Input: part model. Units: mm. Frame: model coordinates. A direction names the side the tool comes from. Round coordinates to 2 decimals unless told otherwise and drop trailing zeros. Loops run counter-clockwise (first coordinate to the right, second up) from the corner with the lowest first, then second, coordinate; pieces in that order, holes last. Notation, with made-up numbers: (-33, -21) -> (25, -21) arc R12 ccw to (25, -15) -> close; hole circle Ø8 at (-2, 26.25). An arc over 180 degrees is marked (long way). Answer as a JSON object with one key per item and string values. Group by question number.
Item 1: Section query B-B on x = -26. Return loops of the section in (y, z), and give its area (3 significant figures).
Item 2: Material intervals for line 1 (Y direction, x = 20.5, z = 4); line 2 (X direction, y = -8, z = 4.25); line 3 (X direction, y = -22.5, z = 17), sorted ascending. Write a range as [from, to].
Item 3: Section query A-A on y = 9. Return loops of the section in (x, z), and give its area (3 significant figures).
Item 4: Draft query along X for faces 3 (the cylindrical face through (-36.19, 29.94, 12.52)), 4 (the cylindrical face through (37.742, 27.501, 12.522)), 5 (the flat face through (0, 29.21, 13)), 6 (the flat face through (0, -29.21, 13)). Return one class per face: released by +X, released by -X, zero draft, split by the parting line, or undercut.
Item 5: Set-up query: faces 1 (the flat face through (-35.56, 1, 13)), 2 (the cylindrical face through (36.19, -29.94, 12.52)). Return all of +Z, -Z, +X, -X, +Y, -Y with unobstructed straight access to the full face (end or side cutting, diameter ignored); none if empty.
from build123d import *

# Parameters (mm, degrees)
F1_DEPTH = 25.4
F2_T     = -2.54
F4_DEPTH = 25.4


with BuildPart() as f1:
    # F0 (on Top) → F1 (new body)
    with BuildSketch(Plane.XY):
        with BuildLine():
            Line((-31.75, -31.75), (31.75, -31.75))
            ThreePointArc((31.75, -31.75), (36.2401280605, -29.8901280605), (38.1, -25.4))
            Line((38.1, -25.4), (38.1, 25.4))
            ThreePointArc((38.1, 25.4), (36.2401280605, 29.8901280605), (31.75, 31.75))
            Line((31.75, 31.75), (-31.75, 31.75))
            ThreePointArc((-31.75, 31.75), (-36.2401280605, 29.8901280605), (-38.1, 25.4))
            Line((-38.1, 25.4), (-38.1, -25.4))
            ThreePointArc((-38.1, -25.4), (-36.2401280605, -29.8901280605), (-31.75, -31.75))
        make_face()
    extrude(amount=F1_DEPTH)

    # F2
    f2_openings = [f1.faces().sort_by_distance(p)[0] for p in [
        (0, 0, 0),
        (0, 0, 25.4),
    ]]
    offset(amount=F2_T, openings=f2_openings)

    # F3 (on Top) → F4 (join)
    with BuildSketch(Plane.XY):
        with BuildLine():
            ThreePointArc((-34.8345838171, 24.6476917684), (-31.3711389564, 22.2476850872), (-28.575, 25.4))
            ThreePointArc((-28.575, 25.4), (-29.2094457266, 27.3042607447), (-30.8592261315, 28.4474820615))
            ThreePointArc((-30.8592261315, 28.4474820615), (-30.7914950358, 28.0740348735), (-30.7688099486, 27.6951738299))
            ThreePointArc((-30.7688099486, 27.6951738299), (-32.0395492039, 25.1546195565), (-34.8345838171, 24.6476917684))
        make_face()
        with BuildLine():
            ThreePointArc((-30.7688099486, 27.6951738299), (-30.7914950358, 28.0740348735), (-30.8592261315, 28.4474820615))
            ThreePointArc((-30.8592261315, 28.4474820615), (-33.9438099486, 27.6951738299), (-34.8345838171, 24.6476917684))
            ThreePointArc((-34.8345838171, 24.6476917684), (-32.0395492039, 25.1546195565), (-30.7688099486, 27.6951738299))
        make_face()
        with BuildLine():
            ThreePointArc((-34.8345838171, 24.6476917684), (-33.9438099486, 27.6951738299), (-30.8592261315, 28.4474820615))
            ThreePointArc((-30.8592261315, 28.4474820615), (-36.1376198972, 29.9903476598), (-34.8345838171, 24.6476917684))
        make_face()
        with BuildLine():
            ThreePointArc((-31.75, -28.575), (-29.5049359697, -27.6450640303), (-28.575, -25.4))
            ThreePointArc((-28.575, -25.4), (-30.5019458319, -22.480584683), (-33.9438099486, -23.1048261701))
            ThreePointArc((-33.9438099486, -23.1048261701), (-31.6987459183, -24.0347621398), (-30.7688099486, -26.2798261701))
            ThreePointArc((-30.7688099486, -26.2798261701), (-31.0243946315, -27.5278803382), (-31.75, -28.575))
        make_face()
        with BuildLine():
            ThreePointArc((-30.7688099486, -26.2798261701), (-31.6987459183, -24.0347621398), (-33.9438099486, -23.1048261701))
            ThreePointArc((-33.9438099486, -23.1048261701), (-34.6968459334, -26.5818308022), (-31.75, -28.575))
            ThreePointArc((-31.75, -28.575), (-31.0243946315, -27.5278803382), (-30.7688099486, -26.2798261701))
        make_face()
        with BuildLine():
            ThreePointArc((-31.75, -28.575), (-34.6968459334, -26.5818308022), (-33.9438099486, -23.1048261701))
            ThreePointArc((-33.9438099486, -23.1048261701), (-36.890655882, -27.4616569723), (-31.75, -28.575))
        make_face()
        with BuildLine():
            ThreePointArc((34.8303002747, 24.630340843), (34.9012361362, 25.0122683738), (34.925, 25.4))
            ThreePointArc((34.925, 25.4), (33.6797927403, 27.9212149808), (30.9208897768, 28.4648329869))
            ThreePointArc((30.9208897768, 28.4648329869), (31.7779499244, 25.4284960104), (34.8303002747, 24.630340843))
        make_face()
        with BuildLine():
            ThreePointArc((30.9208897768, 28.4648329869), (33.6797927403, 27.9212149808), (34.925, 25.4))
            ThreePointArc((34.925, 25.4), (34.9012361362, 25.0122683738), (34.8303002747, 24.630340843))
            ThreePointArc((34.8303002747, 24.630340843), (36.5224050322, 25.7653810896), (37.1761900514, 27.6951738299))
            ThreePointArc((37.1761900514, 27.6951738299), (34.3889216777, 30.8464099661), (30.9208897768, 28.4648329869))
        make_face()
        with BuildLine():
            ThreePointArc((34.8303002747, 24.630340843), (31.7779499244, 25.4284960104), (30.9208897768, 28.4648329869))
            ThreePointArc((30.9208897768, 28.4648329869), (29.526759873, 23.1333221805), (34.8303002747, 24.630340843))
        make_face()
        with BuildLine():
            ThreePointArc((31.8068477454, -28.5744910354), (34.015073574, -27.6248745367), (34.925, -25.4))
            ThreePointArc((34.925, -25.4), (34.6695600543, -24.1522844518), (33.944342306, -23.1053351347))
            ThreePointArc((33.944342306, -23.1053351347), (31.0440156013, -25.1240821363), (31.8068477454, -28.5744910354))
        make_face()
        with BuildLine():
            ThreePointArc((33.944342306, -23.1053351347), (34.6695600543, -24.1522844518), (34.925, -25.4))
            ThreePointArc((34.925, -25.4), (34.015073574, -27.6248745367), (31.8068477454, -28.5744910354))
            ThreePointArc((31.8068477454, -28.5744910354), (35.2489055996, -29.1993862244), (37.1761900514, -26.2798261701))
            ThreePointArc((37.1761900514, -26.2798261701), (36.2260645881, -24.0147525961), (33.944342306, -23.1053351347))
        make_face()
        with BuildLine():
            ThreePointArc((31.8068477454, -28.5744910354), (31.0440156013, -25.1240821363), (33.944342306, -23.1053351347))
            ThreePointArc((33.944342306, -23.1053351347), (28.7928255499, -24.2442559662), (31.8068477454, -28.5744910354))
        make_face()
    extrude(amount=F4_DEPTH)


solid = f1.part
Solved:
{
 "1": {"outline": "(-31.75, 0) -> (-29.21, 0) -> (-29.21, 25.4) -> (-31.75, 25.4) -> close; (29.21, 0) -> (31.75, 0) -> (31.75, 25.4) -> (29.21, 25.4) -> close", "area": "129 mm²"},
 "2": {"line 1": "[-31.75, -29.21], [29.21, 31.75]", "line 2": "[-38.1, -35.56], [35.56, 38.1]", "line 3": "[-38.1, -35.56], [-33.04, -30.46], [30.46, 33.04], [35.56, 38.1]"},
 "3": {"outline": "(-38.1, 0) -> (-35.56, 0) -> (-35.56, 25.4) -> (-38.1, 25.4) -> close; (35.56, 0) -> (38.1, 0) -> (38.1, 25.4) -> (35.56, 25.4) -> close", "area": "129 mm²"},
 "4": {"face 3": "released by -X", "face 4": "released by +X", "face 5": "undercut", "face 6": "undercut"},
 "5": {"face 1": "+Z, -Z", "face 2": "+Z, -Z, +X, -Y"}
}
